```python
from build123d import *

# Parameters (mm, degrees)
F1_DEPTH = 38.1
F2_R     = 11.176
F3_DEPTH = 17.526
F5_D     = 9.652
F7_DEPTH = 3.81
F9_D     = 4.572
F11_D    = 6.35


with BuildPart() as f1:
    # F0 (on Front) → F1 (new body)
    with BuildSketch(Plane.XZ):
        with BuildLine():
            Line((-51.562, 0), (-43.18, -14.732))
            Line((-43.18, -14.732), (-32.8198596835, -14.732))
            Line((-32.8198596835, -14.732), (-32.8198596835, -4.572))
            Line((-32.8198596835, -4.572), (32.4581403165, -4.572))
            Line((32.4581403165, -4.572), (35.814, -14.732))
            Line((35.814, -14.732), (43.942, -14.732))
            Line((43.942, -14.732), (51.562, 0))
            Line((51.562, 0), (51.562, 2.6228378818))
            ThreePointArc((51.562, 2.6228378818), (47.6245523403, 10.89201932), (39.3096618354, 14.732))
            Line((39.3096618354, 14.732), (10.9417002025, 14.732))
            ThreePointArc((10.9417002025, 14.732), (0.0985790513, 25.5751211511), (-10.7445420998, 14.732))
            Line((-10.7445420998, 14.732), (-38.9388203621, 14.732))
            Line((-38.9388203621, 14.732), (-39.1125037328, 14.732))
            ThreePointArc((-39.1125037328, 14.732), (-47.2891089477, 11.676229996), (-51.562, 4.0645938241))
            Line((-51.562, 4.0645938241), (-51.562, 0))
        make_face()
        with BuildLine():
            ThreePointArc((-51.562, 4.0645938241), (-51.7256620474, 2.0322969121), (-51.562, 0))
            Line((-51.562, 0), (-51.562, 4.0645938241))
        make_face()
        with BuildLine():
            ThreePointArc((-38.9388203621, 14.732), (-39.0256620474, 14.7322969121), (-39.1125037328, 14.732))
            Line((-39.1125037328, 14.732), (-38.9388203621, 14.732))
        make_face()
        with BuildLine():
            Line((51.562, 2.6228378818), (51.562, 0))
            ThreePointArc((51.562, 0), (51.6259904882, 1.3114189409), (51.562, 2.6228378818))
        make_face()
    extrude(amount=F1_DEPTH)

    # F2 (on face) → F3 (join)
    with BuildSketch(Plane.XY.offset(14.732)):
        with Locations((0, -11.1125)):
            Circle(F2_R)
    extrude(amount=F3_DEPTH)

    # F5 (through all)
    with Locations(Plane.XY.offset(32.258)):
        with Locations((0, -11.1125)):
            Hole(F5_D / 2)

    # F6 (on face) → F7 (join)
    with BuildSketch(Plane.XY.offset(14.732)):
        with BuildLine():
            Line((10.9417002025, -19.4975990474), (23.3632903546, -19.0058518201))
            ThreePointArc((23.3632903546, -19.0058518201), (29.8632890709, -11.9593614946), (22.8070225567, -5.4699769244))
            Line((22.8070225567, -5.4699769244), (10.9417002025, -5.9754836616))
            Line((10.9417002025, -5.9754836616), (10.9417002025, -8.8360614044))
            ThreePointArc((10.9417002025, -8.8360614044), (11.1172707411, -9.9682678257), (11.176, -11.1125))
            ThreePointArc((11.176, -11.1125), (11.1172707411, -12.2567321743), (10.9417002025, -13.3889385956))
            Line((10.9417002025, -13.3889385956), (10.9417002025, -19.4975990474))
        make_face()
    extrude(amount=F7_DEPTH)

    # F9 (through all)
    with Locations(Plane.XY.offset(18.542)):
        with Locations((23.0953439556, -12.2374957086)):
            Hole(F9_D / 2)

    # F11 (through all)
    with Locations(Plane.XZ.offset(38.1)):
        with Locations((0.0985790513, 14.732)):
            Hole(F11_D / 2)


solid = f1.part
```
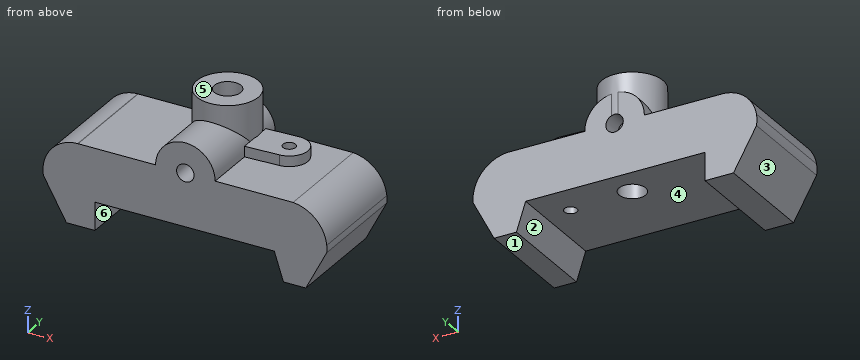
The listing builds one solid part. Answer for the finished solid, in the listing's coordinates (mm). Face numbers are marked on the shaded views. A direction names the side the tool comes from. Round coordinates to 2 decimals unless told otherwise and drop trailing zeros. Order: outer loops, then holes, each group sorted by start corner. A loop starts at its lowest first (then second) coordinate and runs counter-clockwise, first axis right, second up. Notation, with made-up numbers: (12.5, -36.75) - (34.5, -36.75) arc R25 cw to (34.5, 2.25) - close; hole circle Ø3 at (61, 22.5). An arc over 180 degrees is marked (long way). Put each result on its own line as item: value. Start each with the question number.
(1) Find section B-B (z = 23.5). Give the vertices of the cut face in (x, y).
(2) Straight lines are drawn through the part: probe 1 along X at (y, z) = (-10.5, 12.5); probe 2 along Y at (x, z) = (0, 21); probe 3 along Z at (x, y) = (-13, -30). For each, find the intervals that lie inside material, in ascending order. Write a range as from..to.
(3) For the marked faces 5 and 6, determine the directions among +Z, -Z, +X, -X, +Y, -Y from which every point of the face is accessible in a straight line to the end or side of a thin tool.
(4) Find section D-D (x = 26.5). Give the vertices of the cut face in (y, z).
(5) Find section C-C (x = 0). Give the vertices of the cut face in (y, z), plus the area to 3 significant figures.
(6) Determine the mould class of the marked faces 1, 2, 3 and 4 for opening direction X: released by +X, released by -X, zero draft, split by the parting line, or undercut.
(7) Given P1, Ø12, axis at x = 23, z = 5, coming from the +Y side; P2, Ø15.5, axis at x = 25, y = -10, coming from the +Z side; P3, Ø8, axis at y = -14.5, z = 23, coming from the -X side, each flat-ended and moving along its own axis, determine where each tip first touches the part or whether it passes through.
Reply:
1. outline: (-6.28, -38.1) - (6.48, -38.1) - (6.48, -20.22) arc R11.18 ccw to (6.48, -2.01) - (6.48, 0) - (1.19, 0) arc R11.18 ccw to (-1.19, 0) - (-6.28, 0) - (-6.28, -1.87) arc R11.18 ccw to (-6.28, -20.36) - close; hole circle Ø9.65 at (0, -11.11)
2. probe 1: -46.22..-4.79, 4.79..21.61, 24.58..45.66
2. probe 2: -38.1..-15.94, -6.29..0.06
2. probe 3: -4.57..14.73
3. face 5: +Z, +X, -X, +Y, -Y
3. face 6: -Z, +Y, -Y
4. outline: (-38.1, -4.57) - (0, -4.57) - (0, 14.73) - (-6.38, 14.73) - (-6.38, 18.54) - (-18.09, 18.54) - (-18.09, 14.73) - (-38.1, 14.73) - close
5. outline: (-38.1, -4.57) - (-15.94, -4.57) - (-15.94, 11.56) - (-38.1, 11.56) - close; (-38.1, 17.91) - (-15.94, 17.91) - (-15.94, 32.26) - (-22.29, 32.26) - (-22.29, 25.57) - (-38.1, 25.57) - close; (-6.29, -4.57) - (0, -4.57) - (0, 11.56) - (-6.29, 11.56) - close; (-6.29, 17.91) - (0.06, 17.91) - (0.06, 32.26) - (-6.29, 32.26) - close
5. area: 762 mm^2
6. face 1: zero draft
6. face 2: undercut
6. face 3: released by -X
6. face 4: undercut
7. P1: y = 0
7. P2: z = 18.54
7. P3: x = -11.18
